from build123d import *

# Parameters (mm, degrees)
SKETCH_1_R      = 2
SKETCH_1_R_2    = 9.5
SKETCH_1_R_3    = 1.5
SKETCH_1_W      = 4.2
SKETCH_1_H      = 2.2
SKETCH_1_W_2    = 2.2
SKETCH_1_H_2    = 4.2
EXTRUDE_1_DEPTH = 2


with BuildPart() as part:
    # 草图1 → 凸台-拉伸1 (new body)
    with BuildSketch(Plane.XY):
        with BuildLine():
            Line((37.188144312, -134.964533236), (48.99702068, -134.964533236))
            ThreePointArc((48.99702068, -134.964533236), (49.748623267, -130.007441715), (50, -125))
            Line((50, -125), (46.25, -94.741478673))
            Line((46.25, -94.741478673), (24.741807932, -51.739753072))
            Line((24.741807932, -51.739753072), (24.741807932, 0))
            Line((24.741807932, 0), (24.741807932, 37.305457961))
            ThreePointArc((24.741807932, 37.305457961), (30.688954295, 51.663139366), (24.741807932, 66.020820772))
            Line((24.741807932, 66.020820772), (24.741807932, 175))
            ThreePointArc((24.741807932, 175), (0, 199.741807932), (-24.741807932, 175))
            Line((-24.741807932, 175), (-24.741807932, 0))
            Line((-24.741807932, 0), (-24.741807932, -51.739753072))
            Line((-24.741807932, -51.739753072), (-46.25, -94.741478673))
            Line((-46.25, -94.741478673), (-50, -125))
            ThreePointArc((-50, -125), (-49.748623375, -130.007441694), (-48.997021107, -134.964533236))
            Line((-48.997021107, -134.964533236), (-37.188144312, -134.964533236))
            ThreePointArc((-37.188144312, -134.964533236), (-38.041933638, -130.921257055), (-38.457440916, -126.809761925))
            ThreePointArc((-38.457440916, -126.809761925), (-38.5, -125), (-38.457440916, -123.190238075))
            ThreePointArc((-38.457440916, -123.190238075), (-38.457808555, -109.071427319), (-28.474561687, -99.087660532))
            ThreePointArc((-28.474561687, -99.087660532), (-27.223611076, -97.776388924), (-25.912339468, -96.525438313))
            ThreePointArc((-25.912339468, -96.525438313), (-15.928572681, -86.542191445), (-1.809761925, -86.542559084))
            ThreePointArc((-1.809761925, -86.542559084), (0, -86.5), (1.809761925, -86.542559084))
            ThreePointArc((1.809761925, -86.542559084), (15.928572681, -86.542191445), (25.912339468, -96.525438313))
            ThreePointArc((25.912339468, -96.525438313), (27.223611076, -97.776388924), (28.474561687, -99.087660532))
            ThreePointArc((28.474561687, -99.087660532), (38.457808555, -109.071427319), (38.457440916, -123.190238075))
            ThreePointArc((38.457440916, -123.190238075), (38.278220279, -129.126481825), (37.188144312, -134.964533236))
        make_face()
        with Locations((-42.5, -125)):
            Circle(SKETCH_1_R, mode=Mode.SUBTRACT)
        with Locations((-30.0520382, -94.9479618)):
            Circle(SKETCH_1_R, mode=Mode.SUBTRACT)
        with Locations((0, -82.5)):
            Circle(SKETCH_1_R, mode=Mode.SUBTRACT)
        with Locations((30.0520382, -94.9479618)):
            Circle(SKETCH_1_R, mode=Mode.SUBTRACT)
        with Locations((42.5, -125)):
            Circle(SKETCH_1_R, mode=Mode.SUBTRACT)
        with Locations((0, 175)):
            Circle(SKETCH_1_R_2, mode=Mode.SUBTRACT)
        with Locations((0, 192.120903966)):
            Circle(SKETCH_1_R_3, mode=Mode.SUBTRACT)
        with Locations(Location((0, 157.879096034, 0), (0, 0, 180))):
            Circle(SKETCH_1_R_3, mode=Mode.SUBTRACT)
        with Locations((-21.392054648, -28.335407124)):
            Circle(SKETCH_1_R_3, mode=Mode.SUBTRACT)
        with Locations((-21.392054648, 51.664592876)):
            Circle(SKETCH_1_R_3, mode=Mode.SUBTRACT)
        with Locations((-21.392054648, 131.664592876)):
            Circle(SKETCH_1_R_3, mode=Mode.SUBTRACT)
        with Locations((6, 192.120903966)):
            Rectangle(SKETCH_1_W, SKETCH_1_H, mode=Mode.SUBTRACT)
        with BuildLine():
            Line((21.41471253, 49.663139366), (-1.809761925, 49.663139366))
            ThreePointArc((-1.809761925, 49.663139366), (-3.809761925, 51.663139366), (-1.809761925, 53.663139366))
            Line((-1.809761925, 53.663139366), (21.41471253, 53.663139366))
            ThreePointArc((21.41471253, 53.663139366), (23.41471253, 51.663139366), (21.41471253, 49.663139366))
        make_face(mode=Mode.SUBTRACT)
        with Locations((-6, 192.120903966)):
            Rectangle(SKETCH_1_W, SKETCH_1_H, mode=Mode.SUBTRACT)
        with Locations((-21.392054648, 57.664592876)):
            Rectangle(SKETCH_1_W_2, SKETCH_1_H_2, mode=Mode.SUBTRACT)
        with Locations((-6, 157.879096034)):
            Rectangle(SKETCH_1_W, SKETCH_1_H, mode=Mode.SUBTRACT)
        with Locations((6, 157.879096034)):
            Rectangle(SKETCH_1_W, SKETCH_1_H, mode=Mode.SUBTRACT)
        with BuildLine():
            Line((-15, -53.7654447), (-15, 25))
            ThreePointArc((-15, 25), (0, 40), (15, 25))
            Line((15, 25), (15, -53.7654447))
            ThreePointArc((15, -53.7654447), (0, -68.7654447), (-15, -53.7654447))
        make_face(mode=Mode.SUBTRACT)
        with Locations((-21.392054648, -22.335407124)):
            Rectangle(SKETCH_1_W_2, SKETCH_1_H_2, mode=Mode.SUBTRACT)
        with Locations((-21.392054648, -34.335407124)):
            Rectangle(SKETCH_1_W_2, SKETCH_1_H_2, mode=Mode.SUBTRACT)
        with Locations((-21.392054648, 45.664592876)):
            Rectangle(SKETCH_1_W_2, SKETCH_1_H_2, mode=Mode.SUBTRACT)
        with BuildLine():
            Line((-15, 77.43505255), (-15, 132.43505255))
            ThreePointArc((-15, 132.43505255), (0, 147.43505255), (15, 132.43505255))
            Line((15, 132.43505255), (15, 77.43505255))
            ThreePointArc((15, 77.43505255), (0, 62.43505255), (-15, 77.43505255))
        make_face(mode=Mode.SUBTRACT)
        with Locations((-21.392054648, 137.664592876)):
            Rectangle(SKETCH_1_W_2, SKETCH_1_H_2, mode=Mode.SUBTRACT)
        with Locations((-21.392054648, 125.664592876)):
            Rectangle(SKETCH_1_W_2, SKETCH_1_H_2, mode=Mode.SUBTRACT)
    extrude(amount=EXTRUDE_1_DEPTH)


solid = part.part
Verification items for the finished model (mm, model axes). A direction names the side the tool comes from. Coordinates: 2 decimals unless noted, no trailing zeros. Order: outer loops, then holes, each group sorted by start corner. A loop starts at its lowest first (then second) coordinate and runs counter-clockwise, first axis right, second up. Notation, with made-up numbers: M -22.75,83.25 L 5.25,83.25 A7 ccw 5.25,94.25 Z; hole C 65,-32.75 d4. An arc over 180 degrees is marked long. One line per item, written item: value. Start each with the question number.
Item 1: Access from +Z, -Z, +X, -X, +Y, -Y to the whole of each face (thin tool, end or side, straight path). Record for faces 5 (the flat face through (0, 46, 0)), 6 (the flat face through (35.646, -73.542, 0.986)), 7 (the cylindrical face through (0.33, 62.44, 0.99)).
Item 2: Mould release check, pull along Y, two halves, no side actions. Record for faces 1 (the cylindrical face through (-0.33, 147.43, 0.99)), 2 (the cylindrical face through (0.544, 199.736, 0.986)), 3 (the flat face through (0, 46, 2)), 4 (the cylindrical face through (15.741, -86.466, 0.986)): pulls with the +Y half, pulls with the -Y half, needs draft (parallel to the pull), parting line crosses it, or undercut.
Item 3: Depth check by flat-ended pin: P1, Ø0.6, axis at y = 157.5, z = 1, coming from the -X side; P2, Ø1, axis at x = -6.5, z = 1, coming from the +Y side. Enter the tip coordinate at first touch or a pass-through.
Item 4: Sectioned sample at C-C on z = 1.35. Give the number of separate pieces and of enclosed holes in the cut face, then the cut area to 3 significant figures.
Item 5: Thickness scan on probe 1 along Y at (x, z) = (11, 1.5); probe 2 along X at (y, z) = (132.5, 0.1); probe 3 along X at (y, z) = (1, 1.35). Record the ranges inside material, lowest first.
Item 6: Sectioned sample at A-A on y = -4. Record the cut outline in (x, z).
Item 7: Sectioned sample at B-B on x = 18. Record the cut outline in (y, z), then the cut area to 3 significant figures.
Calculated:
1. face 5: -Z, +X, -X, +Y, -Y
1. face 6: +Z, -Z, +X
1. face 7: +Z, -Z
2. face 1: undercut
2. face 2: pulls with the +Y half
2. face 3: needs draft
2. face 4: pulls with the -Y half
3. P1: x = -24.74
3. P2: y = 199
4. separate pieces: 1
4. enclosed holes: 24
4. area: 9,930 mm^2
5. probe 1: -85.26 to -63.96, 35.2 to 49.66, 53.66 to 67.24, 142.63 to 197.16
5. probe 2: -24.74 to -22.64, -20.15 to -15, 15 to 24.74
5. probe 3: -24.74 to -15, 15 to 24.74
6. outline: M -24.74,0 L -15,0 L -15,2 L -24.74,2 Z; M 15,0 L 24.74,0 L 24.74,2 L 15,2 Z
7. outline: M -87.56,0 L 49.66,0 L 49.66,2 L -87.56,2 Z; M 53.66,0 L 191.98,0 L 191.98,2 L 53.66,2 Z
7. area: 551 mm^2
